Can you work these out from the model? Positions are in its coordinate system, mm. Coordinates: 2 decimals unless noted, no trailing zeros. Write each loop counter-clockwise with the first axis right and the second up, starting at its lowest first coordinate (ties: lowest second). Pieces come first, ordered by that corner, then holes. Notation, with made-up numbers: (57.25, -22) - (87.25, -22) arc R21 cw to (87.25, -11) - close; hole circle Ø2 at (53.5, 52.5). An arc over 180 degrees is marked (long way). Use one line per item in the form item = value. Start each with the question number.
(1) If I drill on probe 1 along Y at (x, z) = (9, 1.4) (3 decimals); probe 2 along Y at (x, z) = (89, 1.5); probe 3 along X at (y, z) = (-65.5, 2.95), over which ranges is the centre line in solid material (lowest first)? Write a range as from..to.
(2) For pin 1 Ø1 at (y, z) = (-12, 3) entering from -X; pin 2 Ø4 at (x, y) = (110.57, -56.57) entering from -Z; pin 3 Ø1.2 at (y, z) = (-17.5, 3) entering from +X, each with a flat end and sliding along its axis, tell me the tip position at first contact or that it passes through.
(3) If we section it at A-A on x = 169: Please give me the cut outline in (y, z) (3 decimals).
(4) If we section it at B-B on y = -5: Please give me the cut outline in (x, z) (3 decimals), then the cut area to 3 significant figures.
(5) If we section it at C-C on x = 89: Please give me the cut outline in (y, z), then the cut area to 3 significant figures.
(6) If we section it at D-D on y = -41: Please give me the cut outline in (x, z).
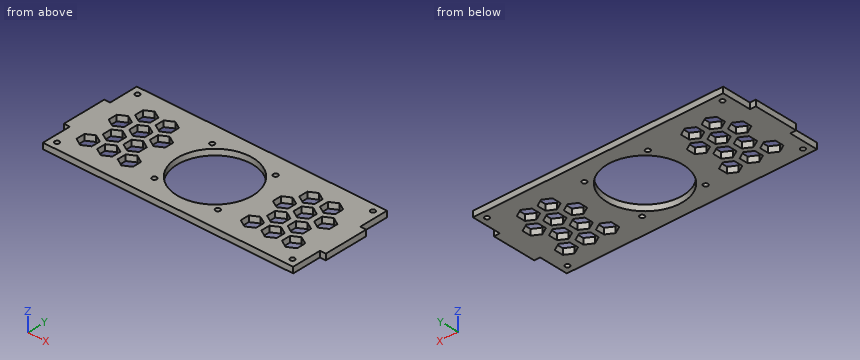
```python
from build123d import *

# Parameters (mm, degrees)
SKETCH_1_W          = 178
SKETCH_1_H          = 70
EXTRUDE_1_DEPTH     = 4
SKETCH_2_R          = 25.75
SKETCH_2_R_2        = 1.575
SKETCH_2_W          = 4
SKETCH_2_H          = 20
CUT_EXTRUDE_1_DEPTH = 192.311264697


with BuildPart() as part:
    # 草图1 → 凸台-拉伸1 (new body)
    with BuildSketch(Plane.XY):
        with Locations((89, -35)):
            Rectangle(SKETCH_1_W, SKETCH_1_H)
    extrude(amount=EXTRUDE_1_DEPTH)

    # 草图2 → 切除-拉伸1 (cut, through all)
    with BuildSketch(Plane.XY.offset(4)):
        with Locations((89, -35)):
            Circle(SKETCH_2_R)
        with Locations((9, -5)):
            Circle(SKETCH_2_R_2)
        with Locations(Location((9, -65, 0), (0, 0, 180))):
            Circle(SKETCH_2_R_2)
        with Locations((169, -65)):
            Circle(SKETCH_2_R_2)
        with Locations(Location((169, -5, 0), (0, 0, 180))):
            Circle(SKETCH_2_R_2)
        with Locations((67.433243174, -13.433243174)):
            Circle(SKETCH_2_R_2)
        with Locations((110.566756826, -13.433243174)):
            Circle(SKETCH_2_R_2)
        with Locations((110.566756826, -56.566756826)):
            Circle(SKETCH_2_R_2)
        with Locations((67.433243174, -56.566756826)):
            Circle(SKETCH_2_R_2)
        with Locations((2, -10)):
            Rectangle(SKETCH_2_W, SKETCH_2_H)
        with Locations((176, -10)):
            Rectangle(SKETCH_2_W, SKETCH_2_H)
        with Locations((176, -60)):
            Rectangle(SKETCH_2_W, SKETCH_2_H)
        with Locations((2, -60)):
            Rectangle(SKETCH_2_W, SKETCH_2_H)
        Polygon((40.196152423, -11), (35, -14), (35, -20), (40.196152423, -23), (45.392304845, -20), (45.392304845, -14), align=None)
        Polygon((26.196152423, -23), (31.392304845, -20), (31.392304845, -14), (26.196152423, -11), (21, -14), (21, -20), align=None)
        Polygon((33.196152423, -35), (38.392304845, -32), (38.392304845, -26), (33.196152423, -23), (28, -26), (28, -32), align=None)
        Polygon((52.392304845, -26), (47.196152423, -23), (42, -26), (42, -32), (47.196152423, -35), (52.392304845, -32), align=None)
        Polygon((24.392304845, -26), (24.392304845, -32), (19.196152423, -35), (14, -32), (14, -26), (19.196152423, -23), align=None)
        Polygon((45.392304845, -38), (45.392304845, -44), (40.196152423, -47), (35, -44), (35, -38), (40.196152423, -35), align=None)
        Polygon((21, -38), (26.196152423, -35), (31.392304845, -38), (31.392304845, -44), (26.196152423, -47), (21, -44), align=None)
        Polygon((14, -56), (19.196152423, -59), (24.392304845, -56), (24.392304845, -50), (19.196152423, -47), (14, -50), align=None)
        Polygon((42, -56), (42, -50), (47.196152423, -47), (52.392304845, -50), (52.392304845, -56), (47.196152423, -59), align=None)
        Polygon((28, -50), (33.196152423, -47), (38.392304845, -50), (38.392304845, -56), (33.196152423, -59), (28, -56), align=None)
        Polygon((144.803847577, -47), (139.607695155, -50), (139.607695155, -56), (144.803847577, -59), (150, -56), (150, -50), align=None)
        Polygon((125.607695155, -56), (130.803847577, -59), (136, -56), (136, -50), (130.803847577, -47), (125.607695155, -50), align=None)
        Polygon((153.607695155, -56), (153.607695155, -50), (158.803847577, -47), (164, -50), (164, -56), (158.803847577, -59), align=None)
        Polygon((137.803847577, -47), (143, -44), (143, -38), (137.803847577, -35), (132.607695155, -38), (132.607695155, -44), align=None)
        Polygon((151.803847577, -35), (146.607695155, -38), (146.607695155, -44), (151.803847577, -47), (157, -44), (157, -38), align=None)
        Polygon((164, -26), (158.803847577, -23), (153.607695155, -26), (153.607695155, -32), (158.803847577, -35), (164, -32), align=None)
        Polygon((136, -26), (136, -32), (130.803847577, -35), (125.607695155, -32), (125.607695155, -26), (130.803847577, -23), align=None)
        Polygon((150, -32), (144.803847577, -35), (139.607695155, -32), (139.607695155, -26), (144.803847577, -23), (150, -26), align=None)
        Polygon((132.607695155, -20), (132.607695155, -14), (137.803847577, -11), (143, -14), (143, -20), (137.803847577, -23), align=None)
        Polygon((157, -20), (151.803847577, -23), (146.607695155, -20), (146.607695155, -14), (151.803847577, -11), (157, -14), align=None)
    extrude(amount=-CUT_EXTRUDE_1_DEPTH, mode=Mode.SUBTRACT)


solid = part.part
```
Reported:
q1.probe_1 = -70..-66.575, -63.425..-6.575, -3.425..0
q1.probe_2 = -70..-60.75, -9.25..0
q1.probe_3 = 4..7.51, 10.49..167.51, 170.49..174
q2.pin_1 = 4
q2.pin_2 = 0
q2.pin_3 = 174
q3.outline = (-70, 0) - (-66.575, 0) - (-66.575, 4) - (-70, 4) - close; (-63.425, 0) - (-6.575, 0) - (-6.575, 4) - (-63.425, 4) - close; (-3.425, 0) - (0, 0) - (0, 4) - (-3.425, 4) - close
q4.outline = (4, 0) - (7.425, 0) - (7.425, 4) - (4, 4) - close; (10.575, 0) - (167.425, 0) - (167.425, 4) - (10.575, 4) - close; (170.575, 0) - (174, 0) - (174, 4) - (170.575, 4) - close
q4.area = 655 mm2
q5.outline = (-70, 0) - (-60.75, 0) - (-60.75, 4) - (-70, 4) - close; (-9.25, 0) - (0, 0) - (0, 4) - (-9.25, 4) - close
q5.area = 74.0 mm2
q6.outline = (0, 0) - (21, 0) - (21, 4) - (0, 4) - close; (31.39, 0) - (35, 0) - (35, 4) - (31.39, 4) - close; (45.39, 0) - (63.96, 0) - (63.96, 4) - (45.39, 4) - close; (114.04, 0) - (132.61, 0) - (132.61, 4) - (114.04, 4) - close; (143, 0) - (146.61, 0) - (146.61, 4) - (143, 4) - close; (157, 0) - (178, 0) - (178, 4) - (157, 4) - close
